Source: CAD feature listing. Evaluate the final solid. Frame: model axes, mm. Face numbers are marked on the shaded views. A direction names the side the tool comes from. Round coordinates to 2 decimals unless told otherwise and drop trailing zeros. Write each loop counter-clockwise with the first axis right and the second up, starting at its lowest first coordinate (ties: lowest second). Pieces come first, ordered by that corner, then holes. Notation, with made-up numbers: (-23.5, 86.25) -> (-16.5, 86.25) arc R27 cw to (-16.5, 107.25) -> close; hole circle Ø4 at (47.5, 87.5). An arc over 180 degrees is marked (long way). Put each result on its own line as item: value.
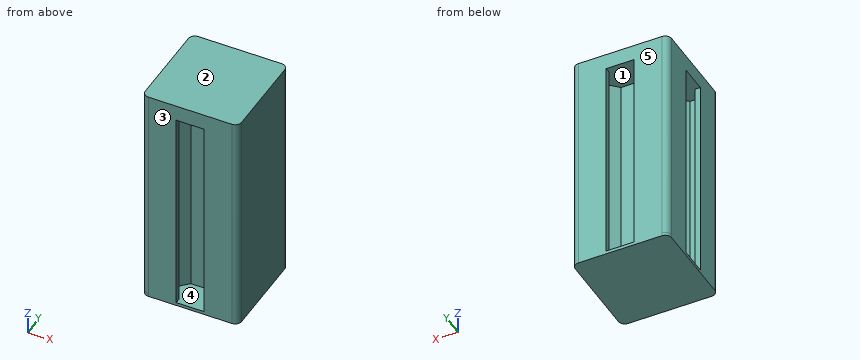
```python
from build123d import *

# Parameters (mm, degrees)
SKETCH1_R                    = 3
SKETCH1_R_2                  = 1.65
BOSS_EXTRUDE1_DEPTH          = 65
FILLET1_R                    = 2
ESTRUSIONE_ESTRUSIONE1_DEPTH = 5
ESTRUSIONE_ESTRUSIONE2_DEPTH = 1
SCHIZZO3_W                   = 65
SCHIZZO3_H                   = 8.7
ESTRUSIONE_ESTRUSIONE3_DEPTH = 1


with BuildPart() as part:
    # Sketch1 → Boss-Extrude1 (new body)
    with BuildSketch(Plane.XY):
        Polygon((-8.46, 9.66), (-4.55, 5.75), (4.55, 5.75), (8.46, 9.66), (8.46, 13.26), (4.35, 13.26), (4.35, 15), (15, 15), (15, 4.35), (13.26, 4.35), (13.26, 8.46), (9.66, 8.46), (5.75, 4.55), (5.75, -4.55), (9.66, -8.46), (13.26, -8.46), (13.26, -4.35), (15, -4.35), (15, -15), (4.35, -15), (4.35, -13.26), (8.46, -13.26), (8.46, -9.59186747), (4.61813253, -5.75), (-4.578313253, -5.75), (-8.420180723, -9.59186747), (-8.420180723, -13.26), (-4.35, -13.26), (-4.35, -15), (-15, -15), (-15, -4.35), (-13.26, -4.35), (-13.26, -8.46), (-9.66, -8.46), (-5.75, -4.55), (-5.75, 4.55), (-9.66, 8.46), (-13.26, 8.46), (-13.26, 4.35), (-15, 4.35), (-15, 15), (-4.35, 15), (-4.35, 13.26), (-8.46, 13.26), align=None)
        Circle(SKETCH1_R, mode=Mode.SUBTRACT)
        with Locations((11.73, 11.73)):
            Circle(SKETCH1_R_2, mode=Mode.SUBTRACT)
        with Locations((11.73, -11.73)):
            Circle(SKETCH1_R_2, mode=Mode.SUBTRACT)
        with Locations((-11.73, -11.73)):
            Circle(SKETCH1_R_2, mode=Mode.SUBTRACT)
        with Locations((-11.73, 11.73)):
            Circle(SKETCH1_R_2, mode=Mode.SUBTRACT)
    extrude(amount=BOSS_EXTRUDE1_DEPTH)

    # Fillet1
    fillet1_edges = [part.edges().sort_by_distance(p)[0] for p in [
        (15, 15, 32.5),
        (15, -15, 32.5),
        (-15, -15, 32.5),
        (-15, 15, 32.5),
    ]]
    fillet(fillet1_edges, radius=FILLET1_R)

    # Schizzo1 → Estrusione-Estrusione1 (add)
    with BuildSketch(Plane.XY.offset(65)):
        with BuildLine():
            Line((13, 15), (4.35, 15))
            Line((4.35, 15), (-4.35, 15))
            Line((-4.35, 15), (-13, 15))
            ThreePointArc((-13, 15), (-14.414213562, 14.414213562), (-15, 13))
            Line((-15, 13), (-15, 4.35))
            Line((-15, 4.35), (-15, -4.35))
            Line((-15, -4.35), (-15, -13))
            ThreePointArc((-15, -13), (-14.414213562, -14.414213562), (-13, -15))
            Line((-13, -15), (-4.35, -15))
            Line((-4.35, -15), (4.35, -15))
            Line((4.35, -15), (13, -15))
            ThreePointArc((13, -15), (14.414213562, -14.414213562), (15, -13))
            Line((15, -13), (15, -4.35))
            Line((15, -4.35), (15, 4.35))
            Line((15, 4.35), (15, 13))
            ThreePointArc((15, 13), (14.414213562, 14.414213562), (13, 15))
        make_face()
    extrude(amount=ESTRUSIONE_ESTRUSIONE1_DEPTH)

    # Schizzo2 → Estrusione-Estrusione2 (add)
    with BuildSketch(Plane(origin=(0, 0, 0), x_dir=(-1, 0, 0), z_dir=(0, 0, -1))):
        with BuildLine():
            Line((-13, 15), (13, 15))
            ThreePointArc((13, 15), (14.414213562, 14.414213562), (15, 13))
            Line((15, 13), (15, -13))
            ThreePointArc((15, -13), (14.414213562, -14.414213562), (13, -15))
            Line((13, -15), (-13, -15))
            ThreePointArc((-13, -15), (-14.414213562, -14.414213562), (-15, -13))
            Line((-15, -13), (-15, 13))
            ThreePointArc((-15, 13), (-14.414213562, 14.414213562), (-13, 15))
        make_face()
    extrude(amount=ESTRUSIONE_ESTRUSIONE2_DEPTH)

    # Schizzo3 → Estrusione-Estrusione3 (add)
    with BuildSketch(Plane(origin=(15, 0, 0), x_dir=(0, 0, -1), z_dir=(1, 0, 0))):
        with Locations((-32.5, 0)):
            Rectangle(SCHIZZO3_W, SCHIZZO3_H)
    extrude(amount=-ESTRUSIONE_ESTRUSIONE3_DEPTH)


solid = part.part
```
Q1. Cut plane C-C on y = 0. Output: boundary loops of the cut face in (x, z), and give its area (4 significant figures).
Ans:
outline: (-15, -1) -> (15, -1) -> (15, 70) -> (-15, 70) -> (-15, 65) -> (-5.75, 65) -> (-5.75, 0) -> (-15, 0) -> close; hole (-3, 0) -> (3, 0) -> (3, 65) -> (-3, 65) -> close; hole (5.75, 0) -> (14, 0) -> (14, 65) -> (5.75, 65) -> close
area: 602.5 mm^2
Q2. Material intervals for line 1 (Y direction, x = 11.73, z = 27.5); line 2 (Z direction, x = 1.5, y = -7); line 3 (X direction, y = -5.25, z = 23.5), sorted ascending. Write a range as [from, to].
Ans:
line 1: y = [-15, -13.38], [-10.08, -8.46], [8.46, 10.08], [13.38, 15]
line 2: z = [-1, 0], [65, 70]
line 3: x = [-15, -13.26], [-6.45, 6.45], [13.26, 15]
Q3. Cut plane A-A on y = -11.73. Output: boundary loops of the cut face in (x, z).
Ans:
outline: (-15, -1) -> (15, -1) -> (15, 70) -> (-15, 70) -> close; hole (-13.38, 0) -> (-10.08, 0) -> (-10.08, 65) -> (-13.38, 65) -> close; hole (-8.42, 0) -> (8.46, 0) -> (8.46, 65) -> (-8.42, 65) -> close; hole (10.08, 0) -> (13.38, 0) -> (13.38, 65) -> (10.08, 65) -> close
Q4. Cut plane B-B on x = 0. Output: boundary loops of the cut face in (y, z), and give its area (4 significant figures).
Ans:
outline: (-15, -1) -> (15, -1) -> (15, 0) -> (5.75, 0) -> (5.75, 65) -> (15, 65) -> (15, 70) -> (-15, 70) -> (-15, 65) -> (-5.75, 65) -> (-5.75, 0) -> (-15, 0) -> close; hole (-3, 0) -> (3, 0) -> (3, 65) -> (-3, 65) -> close
area: 537.5 mm^2
Q5. Pin query (flat end, axial travel): pin 1 (1.4 mm diameter, centred on x = -14, z = 37, fed in from -Y); pin 2 (2.5 mm diameter, centred on x = 0.5, z = 45, fed in from +Y); pin 3 (0.9 mm diameter, centred on y = -14, z = 31.5, fed in from -X). Return the tip coordinate at first contact, or that it passes through.
Ans:
pin 1: stops at y = -14.98
pin 2: stops at y = 5.75
pin 3: stops at x = -14.92
Q6. Cut plane D-D on x = 11.73. Output: boundary loops of the cut face in (y, z).
Ans:
outline: (-15, -1) -> (15, -1) -> (15, 70) -> (-15, 70) -> close; hole (-13.38, 0) -> (-10.08, 0) -> (-10.08, 65) -> (-13.38, 65) -> close; hole (-8.46, 0) -> (8.46, 0) -> (8.46, 65) -> (-8.46, 65) -> close; hole (10.08, 0) -> (13.38, 0) -> (13.38, 65) -> (10.08, 65) -> close
Q7. Reachability of the marked faces 1 and 2 from +Z, -Z, +X, -X, +Y, -Y: full face, straight path, thin tool, end or side. Return the list, or none.
Ans:
face 1: none
face 2: +Z, +X, -X, +Y, -Y
Q8. Draft query along Y for the marked faces 3, 4 and 5. Return one class per face: +Y half, -Y half, draft (parallel to the pull), parting line (faces both ways), or undercut.
Ans:
face 3: -Y half
face 4: undercut
face 5: +Y half
